Could you check a few things on this model? Use its own coordinates, in mm. A direction names the side the tool comes from. Give positions to 0.01 mm unless a question says otherwise; leave off trailing zeros. Write each loop counter-clockwise with the first axis right and the second up, starting at its lowest first coordinate (ties: lowest second). Pieces come first, ordered by that corner, then holes. Notation, with made-up numbers: (85.25, 25) - (129.25, 25) arc R9 ccw to (129.25, 34) - close; hole circle Ø6 at (31.5, 45). An arc over 180 degrees is marked (long way). Answer in a Markdown table with one row per item.
from build123d import *

# Parameters (mm, degrees)
SALIENTE_EXTRUIR1_DEPTH    = 10
CROQUIS3_R                 = 10
CORTAR_EXTRUIR1_DEPTH      = 2
CORTAR_EXTRUIR4_START      = -17
CORTAR_EXTRUIR4_DEPTH      = 34
CORTAR_EXTRUIR5_DEPTH      = 66.741919668
CORTAR_EXTRUIR5_DEPTH_BACK = 10
CROQUIS7_R                 = 2.25
CROQUIS8_R                 = 2.5
CORTAR_EXTRUIR6_DEPTH      = 19
CORTAR_EXTRUIR19_START     = -11
CROQUIS12_R                = 3.5
CORTAR_EXTRUIR19_DEPTH     = 5


# Read off the part's stored shape, not the designer's step: Cortar-Extruir4
with BuildPart() as part:
    # Croquis1 → Saliente-Extruir1 (new body)
    with BuildSketch(Plane(origin=(0, 0, 0), x_dir=(0, 0, -1), z_dir=(1, 0, 0))):
        with BuildLine():
            Line((-15.962347901, 8.291103532), (-9.477641645, 63))
            Line((-9.477641645, 63), (9.477641645, 63))
            Line((9.477641645, 63), (15.962347901, 8.291103532))
            ThreePointArc((15.962347901, 8.291103532), (16.318766271, 5.597695791), (16.748223211, 2.914964711))
            ThreePointArc((16.748223211, 2.914964711), (0, -17), (-16.748223211, 2.914964711))
            ThreePointArc((-16.748223211, 2.914964711), (-16.318766271, 5.597695791), (-15.962347901, 8.291103532))
        make_face()
    extrude(amount=-SALIENTE_EXTRUIR1_DEPTH)

    # Croquis3 → Cortar-Extruir1 (cut)
    with BuildSketch(Plane(origin=(0, 0, 0), x_dir=(0, 0, -1), z_dir=(1, 0, 0))):
        Circle(CROQUIS3_R)
    extrude(amount=-CORTAR_EXTRUIR1_DEPTH, mode=Mode.SUBTRACT)

    # Cortar-Extruir4 outline → Cortar-Extruir4 (cut)
    with BuildSketch(Plane.XY.offset(CORTAR_EXTRUIR4_START)):
        with BuildLine():
            ThreePointArc((0, 13.631567896), (-0.065876274, 10.002392341), (-0.263418304, 6.377998318))
            Line((-0.263418304, 6.377998318), (-1.963636364, -17))
            Line((-1.963636364, -17), (-2.109090909, -19))
            Line((-2.109090909, -19), (0, -19))
            Line((0, -19), (0, 13.631567896))
        make_face()
    extrude(amount=CORTAR_EXTRUIR4_DEPTH, mode=Mode.SUBTRACT)

    # Croquis7 → Cortar-Extruir5 (cut, two sides: drawn at the far end of the back side and taken through both)
    with BuildSketch(Plane(origin=(-2, 0, 0), x_dir=(0, 0, -1), z_dir=(1, 0, 0)).offset(-CORTAR_EXTRUIR5_DEPTH_BACK)):
        with Locations(Location((0, 0, 0), (0, 0, 180))):
            Circle(CROQUIS7_R)
    extrude(amount=CORTAR_EXTRUIR5_DEPTH + CORTAR_EXTRUIR5_DEPTH_BACK, mode=Mode.SUBTRACT)

    # Croquis8 → Cortar-Extruir6 (cut)
    with BuildSketch(Plane(origin=(0, 0, 0), x_dir=(1, 0, 0), z_dir=(0, 1, 0))):
        with Locations(Location((-6, 0, 0), (0, 0, 270))):
            Circle(CROQUIS8_R)
    extrude(amount=-CORTAR_EXTRUIR6_DEPTH, mode=Mode.SUBTRACT)

    # Croquis12 → Cortar-Extruir19 (cut)
    with BuildSketch(Plane(origin=(0, 0, 0), x_dir=(1, 0, 0), z_dir=(0, 1, 0)).offset(CORTAR_EXTRUIR19_START)):
        with Locations(Location((-6, 0, 0), (0, 0, 270))):
            Circle(CROQUIS12_R)
    extrude(amount=-CORTAR_EXTRUIR19_DEPTH, mode=Mode.SUBTRACT)


solid = part.part
1) Will these pins go through, and if not, where does the flat tip stop? P1, Ø3, axis at x = -4, z = 7.5, coming from the -Y side; P2, Ø2, axis at x = -4.5, z = 1, coming from the -Y side; P3, Ø16, axis at y = 0.5, z = 4.5, coming from the +X side.
Check values:
| item | result |
|---|---|
| P1 | stops at y = -15.91 |
| P2 | stops at y = -16.99 |
| P3 | stops at x = -0.13 |
2) Imagine slicing it at B-B (x = -6). List the corners of the cut face in (y, z) for me, then the cut area to 3 significant figures.
Check values:
| item | result |
|---|---|
| outline | (-16.82, -2.5) arc R17 ccw to (2.91, -16.75) arc R100 cw to (8.29, -15.96) - (63, -9.48) - (63, 9.48) - (8.29, 15.96) arc R100 cw to (2.91, 16.75) arc R17 ccw to (-16.82, 2.5) - (-16, 2.5) - (-16, 3.5) - (-11, 3.5) - (-11, 2.5) - (0, 2.5) - (0, 2.25) arc R2.25 cw to (0, -2.25) - (0, -2.5) - (-11, -2.5) - (-11, -3.5) - (-16, -3.5) - (-16, -2.5) - close |
| area | 2,020 mm2 |
3) We'd pull the mould along Z, two halves only. Please class faces 5 (the face through (-1.48, -10.34, -0.24)), 6 (the face through (-3, -17, 0)), 7 (the face through (-8, -16, 2)): +Z half, -Z half, draft (parallel to the pull), parting line (faces both ways), or undercut.
Check values:
| item | result |
|---|---|
| face 5 | draft |
| face 6 | parting line |
| face 7 | undercut |
4) On a 3-axis mill with a long thin cutter (end or side, diameter ignored), from which of +Z, -Z, +X, -X, +Y, -Y can I reach the whole of each face in a straight line? I mean faces 1 (the face through (-8, -11, 2)), 2 (the face through (-1.234, 9.915, 1.302)), 3 (the face through (-5.249, -16.496, 2.385)), 4 (the face through (0, 39, 0)). Say none if no direction works.
Check values:
| item | result |
|---|---|
| face 1 | none |
| face 2 | +X |
| face 3 | -Y |
| face 4 | +Z, -Z, +X, +Y, -Y |
5) Imagine slicing it at A-A (z = 0). List the corners of the cut face in (x, y) for me, then the cut area to 3 significant figures.
Check values:
| item | result |
|---|---|
| outline | (-10, -17) - (-8.5, -17) - (-8.5, -16) - (-9.5, -16) - (-9.5, -11) - (-8.5, -11) - (-8.5, -2.25) - (-10, -2.25) - close; (-10, 2.25) - (-2, 2.25) - (-2, 10) - (-0.07, 10) arc R100 ccw to (0, 13.63) - (0, 63) - (-10, 63) - close; (-3.5, -17) - (-1.96, -17) - (-1.45, -10) - (-2, -10) - (-2, -2.25) - (-3.5, -2.25) - (-3.5, -11) - (-2.5, -11) - (-2.5, -16) - (-3.5, -16) - close |
| area | 628 mm2 |
6) If I drill on line 1 (X direction, y = -7.25, z = 0); line 2 (Z direction, x = -6, y = -5); line 3 (X direction, y = -6, z = 2), over which ranges is the centre line in solid material (lowest first)?
Check values:
| item | result |
|---|---|
| line 1 | x = -10 to -8.5, -3.5 to -2 |
| line 2 | z = -16.25 to -2.5, 2.5 to 16.25 |
| line 3 | x = -10 to -7.5, -4.5 to -2 |
7) Imagine slicing it at C-C (z = 11.5). List the corners of the cut face in (x, y) for me, then the cut area to 3 significant figures.
Check values:
| item | result |
|---|---|
| outline | (-10, -12.52) - (-1.64, -12.52) - (-0.26, 6.38) arc R100 ccw to (0, 13.63) - (0, 45.94) - (-10, 45.94) - close |
| area | 566 mm2 |
8) Imagine slicing it at D-D (y = 46.5). List the corners of the cut face in (x, z) for me, then the cut area to 3 significant figures.
Check values:
| item | result |
|---|---|
| outline | (-10, -11.43) - (0, -11.43) - (0, 11.43) - (-10, 11.43) - close |
| area | 229 mm2 |
